from build123d import *

# Parameters (mm, degrees)
SKETCH1_W           = 6.35
SKETCH1_H           = 6.35
BOSS_EXTRUDE1_DEPTH = 6.35


with BuildPart() as part:
    # Sketch1 → Boss-Extrude1 (new body)
    with BuildSketch(Plane(origin=(0, 0, 0), x_dir=(1, 0, 0), z_dir=(0, 1, 0))):
        Polygon((-76.2, -38.1), (-76.2, -63.5), (-69.85, -63.5), (-63.5, -63.5), (-63.5, -69.85), (-63.5, -76.2), (-38.1, -76.2), (-38.1, -69.85), (-31.75, -69.85), (-31.75, -76.2), (31.75, -76.2), (31.75, -69.85), (38.1, -69.85), (38.1, -76.2), (63.5, -76.2), (63.5, -69.85), (63.5, -63.5), (69.85, -63.5), (76.2, -63.5), (76.2, -38.1), (69.85, -38.1), (69.85, -31.75), (76.2, -31.75), (76.2, 31.75), (69.85, 31.75), (69.85, 38.1), (76.2, 38.1), (76.2, 63.5), (69.85, 63.5), (63.5, 63.5), (63.5, 69.85), (63.5, 76.2), (38.1, 76.2), (38.1, 69.85), (31.75, 69.85), (31.75, 76.2), (-31.75, 76.2), (-31.75, 69.85), (-38.1, 69.85), (-38.1, 76.2), (-63.5, 76.2), (-63.5, 69.85), (-63.5, 63.5), (-69.85, 63.5), (-76.2, 63.5), (-76.2, 38.1), (-69.85, 38.1), (-69.85, 31.75), (-76.2, 31.75), (-76.2, -31.75), (-69.85, -31.75), (-69.85, -38.1), align=None)
        with Locations((-66.675, -66.675)):
            Rectangle(SKETCH1_W, SKETCH1_H)
        with Locations((66.675, -66.675)):
            Rectangle(SKETCH1_W, SKETCH1_H)
        with Locations((66.675, 66.675)):
            Rectangle(SKETCH1_W, SKETCH1_H)
        with Locations((-66.675, 66.675)):
            Rectangle(SKETCH1_W, SKETCH1_H)
    extrude(amount=BOSS_EXTRUDE1_DEPTH)


solid = part.part
Work out the finished part from the listing and answer in its coordinate system (mm). A direction names the side the tool comes from. Round coordinates to 2 decimals unless told otherwise and drop trailing zeros. Order: outer loops, then holes, each group sorted by start corner. A loop starts at its lowest first (then second) coordinate and runs counter-clockwise, first axis right, second up. Notation, with made-up numbers: M -33.5,-12.5 L -21.5,-12.5 A13 cw -21.5,-7.5 Z; hole C 67,17.25 d5. An arc over 180 degrees is marked long. Put each result on its own line as item: value. Start each with the question number.
Q1. A straight line is drawn through the part: L1, parallel to Z at x = -37, y = 5. Find the intervals that lie inside material, in ascending order. Write a range as [from, to].
Q2. A tool of negligible diameter and unlimited length cuts with its end or side. For faces 1 (the flat face through (-67, 3, 69.85)), 2 (the flat face through (31.75, 3, 73)), 3 (the flat face through (-35, 3, -69.85)), 4 (the flat face through (69.85, 3, -35)), 5 (the flat face through (63.5, 3, 73)), from which of +Z, -Z, +X, -X, +Y, -Y can it reach the whole face along a straight path? Write none if from no direction.
Q3. For a pull along X with two mould halves and no side action, classify faces 6 (the flat face through (73, 3, 63.5)), 7 (the flat face through (-31.75, 3, -73)), 8 (the flat face through (-63.5, 3, 73)) as pulls with the +X half, pulls with the -X half, needs draft (parallel to the pull), parting line crosses it, or undercut.
Q4. Flat-ended cylindrical pins translate along their axes: pin 1 (3 mm diameter, centred on y = 2, z = -74.5, fed in from +X); pin 2 (1.9 mm diameter, centred on x = 33.5, y = 3, fed in from +Z); pin 3 (1.9 mm diameter, centred on x = -72, y = 2, fed in from +Z). Find the tip coordinate at first contact, or state that the pin passes through.
Q5. Section A-A, the plane z = -66.5 is taken. Write down the section's boundary in (x, y), and give its area (3 significant figures).
Findings below:
1. L1: z = [-69.85, 69.85]
2. face 1: +Z, -X, +Y, -Y
2. face 2: +Z, +Y, -Y
2. face 3: -Z, +Y, -Y
2. face 4: +X, +Y, -Y
2. face 5: +Z, +X, +Y, -Y
3. face 6: needs draft
3. face 7: undercut
3. face 8: pulls with the -X half
4. pin 1: stops at x = 63.5
4. pin 2: stops at z = 69.85
4. pin 3: stops at z = 63.5
5. outline: M -69.85,0 L 69.85,0 L 69.85,6.35 L -69.85,6.35 Z
5. area: 887 mm^2
